Verification items for this drawing (mm, ordinates from the low corner). Give positions to 0.01 mm unless a question says otherwise; leave off trailing zeros. Loops run counter-clockwise (first coordinate to the right, second up) from the corner with the lowest first, then second, coordinate; pieces in that order, holes last. Notation, with made-up numbers: (-29.5, 86.5) -> (10.5, 86.5) arc R15 cw to (10.5, 92.5) -> close; hole circle Ø9 at (52.5, 58). An arc over 180 degrees is marked (long way). Write item = value, one per line.
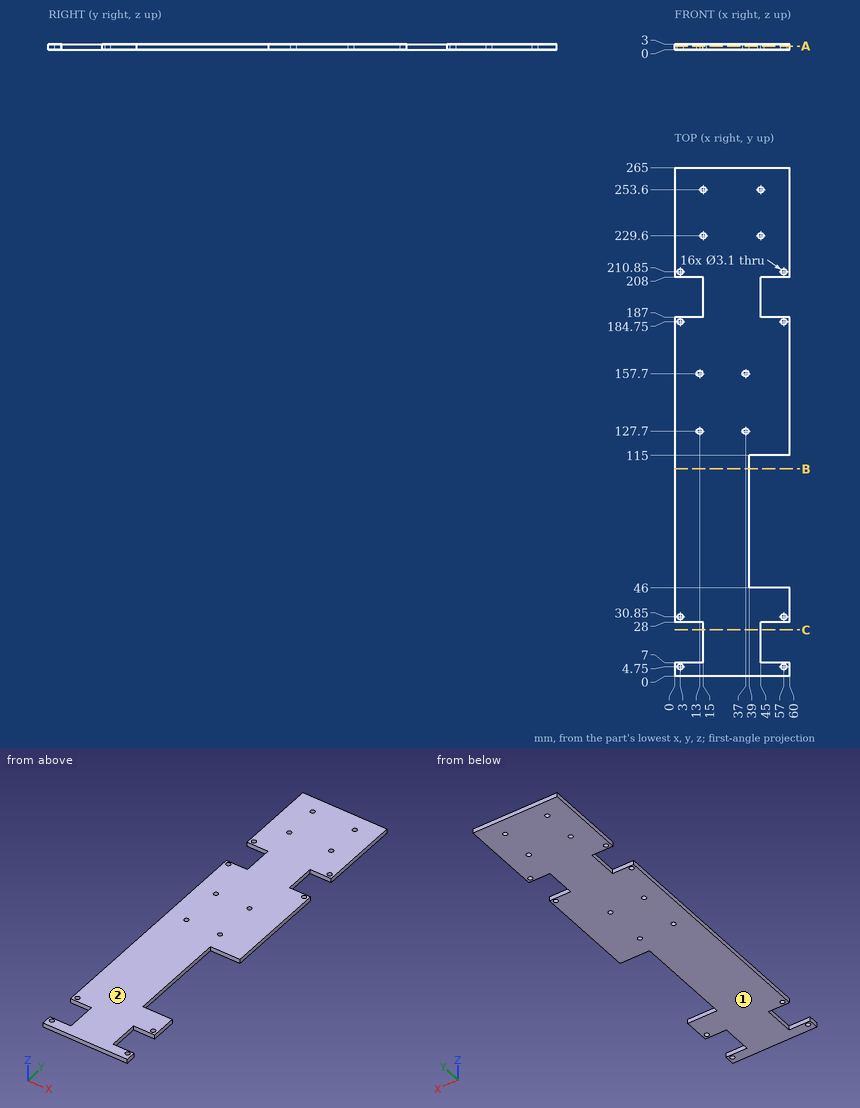
Item 1: Section check A-A, the plane z = 1.9. Give the number of separate pieces and of enclosed holes in the cut face, plus the area to 3 significant figures.
Answer:
separate_pieces = 1
enclosed_holes = 16
area = 13,100 mm^2
Item 2: Section check C-C, the plane y = 24. Record the cut outline in (x, z), plus the area to 3 significant figures.
Answer:
outline = (15, 0) -> (45, 0) -> (45, 3) -> (15, 3) -> close
area = 90.0 mm^2
Item 3: Thickness scan on L1, parallel to Y at x = 37, z = 1.8; L2, parallel to Y at x = 47.5, z = 1.35; L3, parallel to X at y = 253.6, z = 2.2. Record the ranges inside material, lowest first. Write a range as [from, to].
Answer:
L1 = [0, 126.15], [129.25, 156.15], [159.25, 265]
L2 = [0, 7], [28, 46], [115, 187], [208, 265]
L3 = [0, 13.45], [16.55, 43.45], [46.55, 60]
Item 4: Draft check along Z on the marked faces 1 and 2. Enter one of: +Z half, -Z half, draft (parallel to the pull), parting line (faces both ways), or undercut.
Answer:
face_1 = -Z half
face_2 = +Z half
Item 5: Section check B-B, the plane y = 108. Record the cut outline in (x, z), plus the area to 3 significant figures.
Answer:
outline = (0, 0) -> (39, 0) -> (39, 3) -> (0, 3) -> close
area = 117 mm^2
